Part model, mm, in its own coordinate system. A direction names the side the tool comes from. Give positions to 0.01 mm unless a question says otherwise; leave off trailing zeros. Order: outer loops, then holes, each group sorted by start corner. A loop starts at its lowest first (then second) coordinate and runs counter-clockwise, first axis right, second up. Notation, with made-up numbers: (-10, -5) - (-5, -5) arc R24 ccw to (-5, 31) - close; hole circle Ø1 at (66, 57.5). An arc over 180 degrees is marked (long way). Use a Markdown table: item, result. Add a question column.
from build123d import *

# Parameters (mm, degrees)
SKETCH1_R           = 150
BOSS_EXTRUDE1_DEPTH = 500
SKETCH2_R           = 150
SKETCH2_R_2         = 90
CUT_EXTRUDE1_DEPTH  = 70
SKETCH4_R           = 67.5
BOSS_EXTRUDE2_DEPTH = 350
SKETCH5_R           = 150
CUT_EXTRUDE3_DEPTH  = 100
SKETCH6_R           = 90
CUT_EXTRUDE4_DEPTH  = 401.0000001


with BuildPart() as part:
    # Sketch1 → Boss-Extrude1 (new body)
    with BuildSketch(Plane(origin=(0, 0, 0), x_dir=(1, 0, 0), z_dir=(0, 1, 0))):
        Circle(SKETCH1_R)
    extrude(amount=BOSS_EXTRUDE1_DEPTH)

    # Sketch2 → Cut-Extrude1 (cut)
    with BuildSketch(Plane.XZ):
        Circle(SKETCH2_R)
        Circle(SKETCH2_R_2, mode=Mode.SUBTRACT)
    extrude(amount=-CUT_EXTRUDE1_DEPTH, mode=Mode.SUBTRACT)

    # Sketch4 → Boss-Extrude2 (add)
    with BuildSketch(Plane.XY):
        with Locations((0, 249.430268714)):
            Circle(SKETCH4_R)
    extrude(amount=BOSS_EXTRUDE2_DEPTH)

    # Sketch5 → Cut-Extrude3 (cut)
    with BuildSketch(Plane(origin=(0, 500, 0), x_dir=(1, 0, 0), z_dir=(0, 1, 0))):
        Circle(SKETCH5_R)
    extrude(amount=-CUT_EXTRUDE3_DEPTH, mode=Mode.SUBTRACT)

    # Sketch6 → Cut-Extrude4 (cut, through all)
    with BuildSketch(Plane.XZ):
        Circle(SKETCH6_R)
    extrude(amount=-CUT_EXTRUDE4_DEPTH, mode=Mode.SUBTRACT)


solid = part.part
1. Cut at D-D (y = 332). Write the cut outline in (x, z), plus the area to 3 significant figures.
2. Cut at A-A (x = 0). Write the cut outline in (y, z), plus the area to 3 significant figures.
3. Mould opens along Z. For faces 3 (the face through (-1, 250, 350)), 4 (the face through (65, 70, -65)), 5 (the face through (41.53, 232.69, -79.845)), 6 (the face through (-19.527, 232.69, -148.724)) say: released by +Z, released by -Z, zero draft, split by the parting line, or undercut.
4. Pin check, flat tips, straight feed: P1, Ø5, axis at y = 332.5, z = 113.5, coming from the -X side; P2, Ø10, axis at y = 168.5, z = 49.5, coming from the +X side; P3, Ø2, axis at x = 116.5, y = 364, coming from the +Z side. Stop position of each tip, or through.
5. Cut at C-C (z = -67). Write the cut outline in (x, y), plus the area to 3 significant figures.
6. Tool access for faces 1 (the face through (65, 400, 65)), 2 (the face through (-67.435, 252.398, 240.465)): list every direction of +Z, -Z, +X, -X, +Y, -Y with a clear straight run to the whole face (end or side of a thin tool).
7. Cut at B-B (z = 0). Write the cut outline in (x, y), plus the area to 3 significant figures.
8. Drill centre lines: probe 1 along Z at (x, y) = (0, 159.5); probe 2 along Z at (x, y) = (0, 275); probe 3 along X at (y, z) = (129, -39). Where is each one in solid material? Low to high. Write a range as [from, to].
Responses:
| question | item | result |
|---|---|---|
| 1 | outline | circle Ø300 at (0, 0); hole circle Ø180 at (0, 0) |
| 1 | area | 45,200 mm² |
| 2 | outline | (70, -150) - (400, -150) - (400, -90) - (70, -90) - close; (70, 90) - (400, 90) - (400, 150) - (316.93, 150) - (316.93, 350) - (181.93, 350) - (181.93, 150) - (70, 150) - close |
| 2 | area | 66,600 mm² |
| 3 | face 3 | released by +Z |
| 3 | face 4 | zero draft |
| 3 | face 5 | undercut |
| 3 | face 6 | split by the parting line |
| 4 | P1 | stops at x = -100.89 |
| 4 | P2 | stops at x = 143.25 |
| 4 | P3 | stops at z = 95.71 |
| 5 | outline | (-134.21, 70) - (-60.09, 70) - (-60.09, 400) - (-134.21, 400) - close; (60.09, 70) - (134.21, 70) - (134.21, 400) - (60.09, 400) - close |
| 5 | area | 48,900 mm² |
| 6 | face 1 | +Z, -Z, +X, -X, +Y |
| 6 | face 2 | +Z |
| 7 | outline | (-150, 70) - (-90, 70) - (-90, 400) - (-150, 400) - close; (90, 70) - (150, 70) - (150, 400) - (90, 400) - close |
| 7 | area | 39,600 mm² |
| 8 | probe 1 | z = [-150, -90], [90, 150] |
| 8 | probe 2 | z = [-150, -90], [90, 350] |
| 8 | probe 3 | x = [-144.84, -81.11], [81.11, 144.84] |
